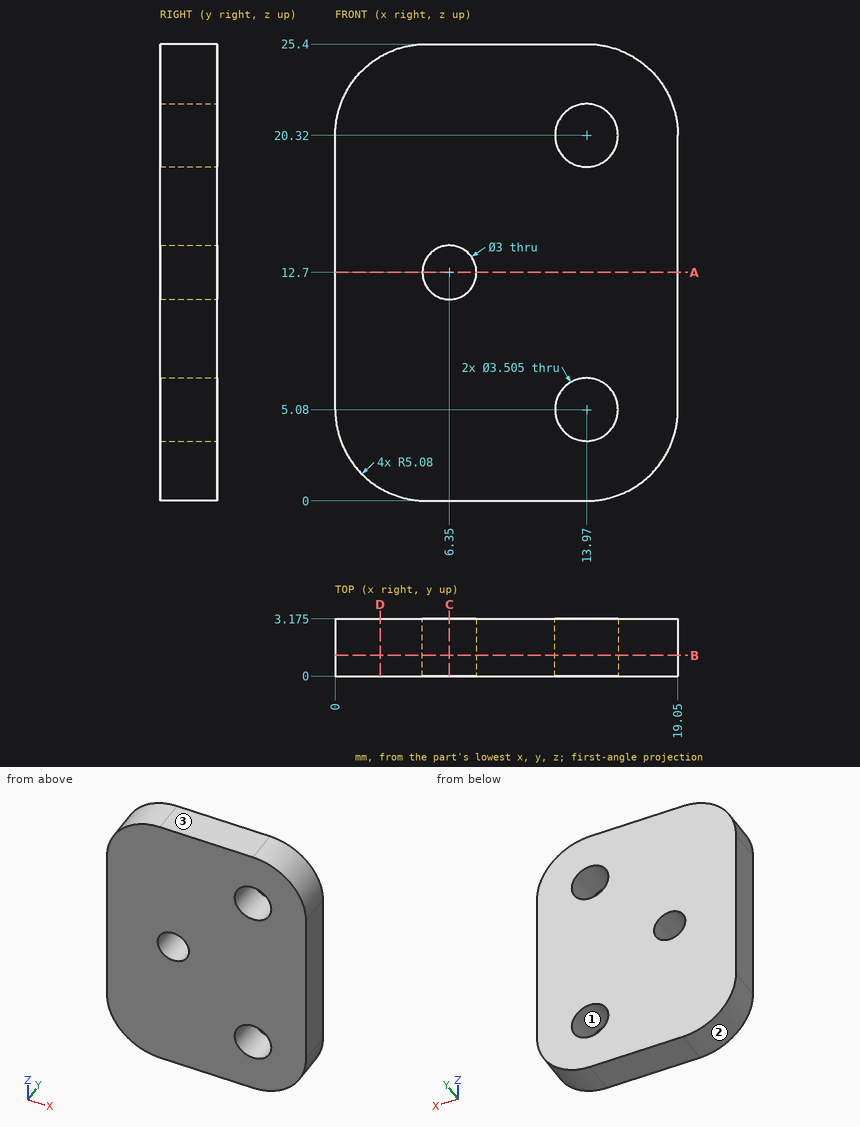
Study the drawing (mm; zero at the part's minimum x, y, z) and answer. Give positions to 0.01 mm unless a question says otherwise; leave off trailing zeros. Loops run counter-clockwise (first coordinate to the right, second up) from the corner with the lowest first, then second, coordinate; pieces in that order, holes last. Notation, with made-up numbers: M 30.25,-12.5 L 77.25,-12.5 A21 ccw 77.25,18.5 Z; hole C -28.75,66 d10. An arc over 180 degrees is marked long. Use CSV: the item, a comma, the result in double quotes.
1) Find section D-D on x = 2.5. Write down the section's boundary in (y, z) (3 decimals).
Answer:
outline,"M 0,0.704 L 3.175,0.704 L 3.175,24.696 L 0,24.696 Z"
2) Given P1, Ø2.5, axis at x = 6.35, z = 12.7, coming from the +Y side, flat-ended and moving along its own axis, determine where the tip first touches the part or whether it passes through.
Answer:
P1,"through"
3) Find section B-B on y = 1.15. Give the number of separate pieces and of enclosed holes in the cut face, plus the area to 3 significant figures.
Answer:
separate pieces,"1"
enclosed holes,"3"
area,"435 mm^2"
4) Consider L1, parallel to Z at x = 6.35, y = 1.75; L2, parallel to Z at x = 14.75, y = 2.5; L3, parallel to X at y = 1.8, z = 19.75. Determine where each line is inside the solid, lowest interval first.
Answer:
L1,"0 to 11.2, 14.2 to 25.4"
L2,"0.06 to 3.51, 6.65 to 18.75, 21.89 to 25.34"
L3,"0 to 12.31, 15.63 to 19.05"
5) Determine the mould class of the marked faces 1, 2 and 3 for opening direction Z: released by +Z, released by -Z, zero draft, split by the parting line, or undercut.
Answer:
face 1,"undercut"
face 2,"released by -Z"
face 3,"released by +Z"
6) Find section C-C on x = 6.35. Write down the section's boundary in (y, z) (3 decimals).
Answer:
outline,"M 0,0 L 3.175,0 L 3.175,11.2 L 0,11.2 Z; M 0,14.2 L 3.175,14.2 L 3.175,25.4 L 0,25.4 Z"
7) Find section A-A on z = 12.7. Write down the section's boundary in (x, y) (3 decimals).
Answer:
outline,"M 0,0 L 4.85,0 L 4.85,3.175 L 0,3.175 Z; M 7.85,0 L 19.05,0 L 19.05,3.175 L 7.85,3.175 Z"
